Source: three-view drawing plus pictorial views. Frame: mm from the lowest corner of the part. Round coordinates to 2 decimals unless told otherwise and drop trailing zeros. Write each loop counter-clockwise with the first axis right and the second up, starting at its lowest first coordinate (ties: lowest second). Pieces come first, ordered by that corner, then holes.
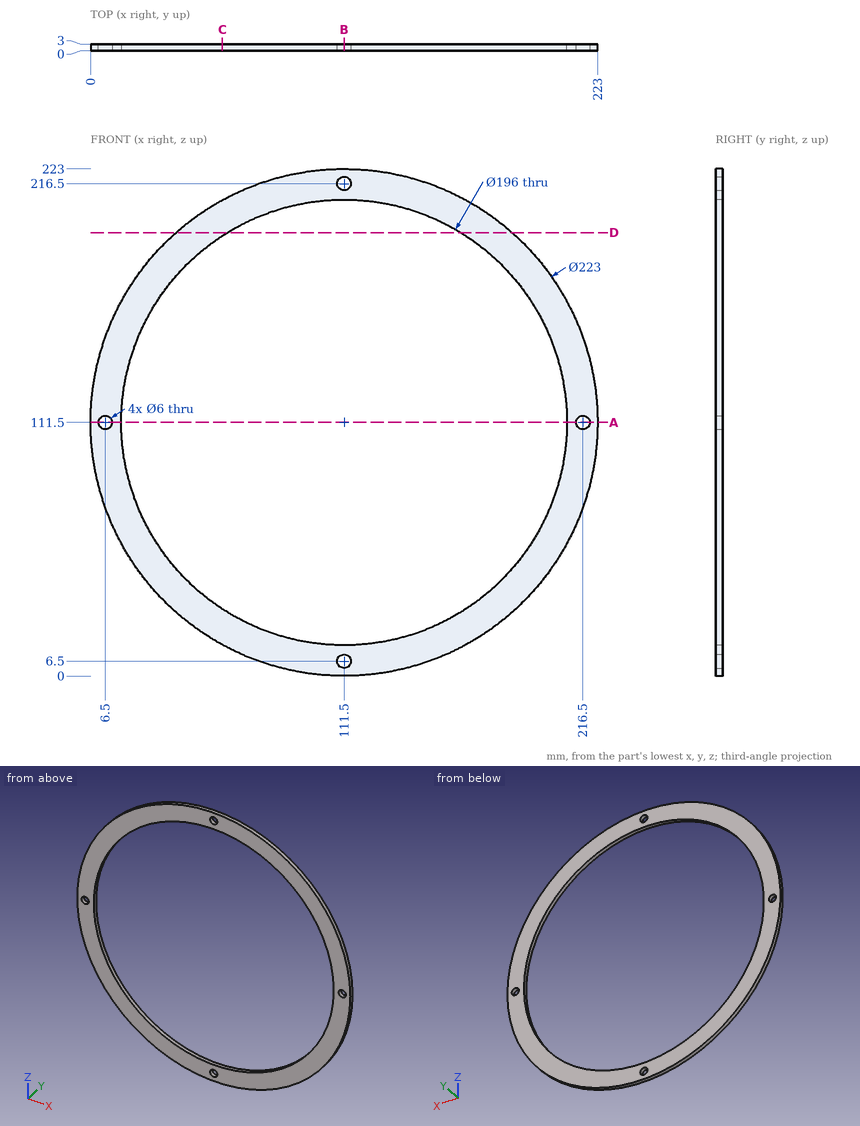
1) Section C-C on x = 58. Output: boundary loops of the cut face in (y, z), plus the area to 3 significant figures.
2) Line query: probe 1 along Z at (x, y) = (111.5, 1.1); probe 2 along Z at (x, y) = (23.5, 0.85). Output: solid intervals per line, ascending.
3) Section B-B on x = 111.5. Output: boundary loops of the cut face in (y, z), plus the area to 3 significant figures.
4) First-contact query: P1, Ø1, axis at y = 1.5, z = 102, coming from the +X side; P2, Ø1.5, axis at x = 157, y = 0.5, coming from the +Z side; P3, Ø5, axis at x = 6.5, z = 111.5, coming from the +Y side. Flat tips, straight axial feed; report the tip coordinate or a pass-through.
5) Section A-A on z = 111.5. Output: boundary loops of the cut face in (x, y), plus the area to 3 significant figures.
6) Section D-D on z = 195. Output: boundary loops of the cut face in (x, y).
Filled in:
1. outline: (0, 13.67) - (3, 13.67) - (3, 29.39) - (0, 29.39) - close; (0, 193.61) - (3, 193.61) - (3, 209.33) - (0, 209.33) - close
1. area: 94.3 mm2
2. probe 1: z = 0 to 3.5, 9.5 to 13.5, 209.5 to 213.5, 219.5 to 223
2. probe 2: z = 43.03 to 68.37, 154.63 to 179.97
3. outline: (0, 0) - (3, 0) - (3, 3.5) - (0, 3.5) - close; (0, 9.5) - (3, 9.5) - (3, 13.5) - (0, 13.5) - close; (0, 209.5) - (3, 209.5) - (3, 213.5) - (0, 213.5) - close; (0, 219.5) - (3, 219.5) - (3, 223) - (0, 223) - close
3. area: 45.0 mm2
4. P1: stops at x = 222.64
4. P2: stops at z = 213.63
4. P3: passes through
5. outline: (0, 0) - (3.5, 0) - (3.5, 3) - (0, 3) - close; (9.5, 0) - (13.5, 0) - (13.5, 3) - (9.5, 3) - close; (209.5, 0) - (213.5, 0) - (213.5, 3) - (209.5, 3) - close; (219.5, 0) - (223, 0) - (223, 3) - (219.5, 3) - close
5. area: 45.0 mm2
6. outline: (37.61, 0) - (60.2, 0) - (60.2, 3) - (37.61, 3) - close; (162.8, 0) - (185.39, 0) - (185.39, 3) - (162.8, 3) - close
